Design review of the part built by this model. Coordinates are the model's own, in mm. Face numbers are marked on the shaded views. A direction names the side the tool comes from. Coordinates: 2 decimals unless noted, no trailing zeros. Loops run counter-clockwise (first coordinate to the right, second up) from the corner with the lowest first, then second, coordinate; pieces in that order, holes last. Notation, with made-up numbers: (78, 52) - (112, 52) arc R21 ccw to (112, 62) - close; hole circle Ø9 at (32, 72.5). An arc over 180 degrees is marked (long way). Answer in a Markdown table with one row per item. Add a question column.
(1) The part is to be moulded in two halves that separate along Y. For the marked faces 6, 7 and 8, say which applies: released by +Y, released by -Y, zero draft, split by the parting line, or undercut.
(2) For the marked faces 1, 2, 3, 4 and 5, list the 3-axis set-ups (+Z, -Z, +X, -X, +Y, -Y) from which the entire face can be reached by the end or side of a thin tool; tool diameter is ignored.
(3) Clearance check with flat-ended pins moving along their axes: pin 1 (1.9 mm diameter, centred on x = -0.5, y = 2, fed in from +Z); pin 2 (0.6 mm diameter, centred on x = 43, y = 31.5, fed in from +Z) (3 decimals); pin 3 (3.5 mm diameter, centred on x = 44.25, z = 4.625, fed in from +Y); pin 4 (1.6 mm diameter, centred on x = -4.5, y = 31.5, fed in from -Z) (3 decimals). State where each tip first meets the part, or that it passes through.
(4) We need section C-C, the plane x = 44.25. Write out the cut boundary in (y, z) (3 decimals).
(5) We need section A-A, the plane x = 31.5. Write out the cut boundary in (y, z), plus the area to 3 significant figures.
(6) We need section B-B, the plane y = 18. Write out the cut boundary in (x, z), plus the area to 3 significant figures.
(7) We need section D-D, the plane x = 9.35. Write out the cut boundary in (y, z) (3 decimals).
(8) To check wall thickness, follow L1, parallel to Z at x = 44, y = 29; L2, parallel to X at y = 30, z = 6.5; L3, parallel to Y at x = 16, z = 3.25. State the ranges of each line that lie inside material, in increasing order. Write a range as [from, to].
from build123d import *

# Parameters (mm, degrees)
SKETCH1_W                 = 40
SKETCH1_H                 = 20
BOSS_EXTRUDE1_DEPTH       = 34.4
BOSS_EXTRUDE2_DEPTH       = 2.8
SKETCH4_R                 = 6.95
BOSS_EXTRUDE3_DEPTH       = 1.7
SKETCH5_R                 = 5.075
BOSS_EXTRUDE4_DEPTH       = 0.5
SKETCH6_R                 = 2.875
BOSS_EXTRUDE5_DEPTH       = 3.25
BOSS_EXTRUDE6_DEPTH       = 0.75
SKETCH8_W                 = 20
SKETCH8_H                 = 2.5
BOSS_EXTRUDE7_DEPTH       = 6.7
SKETCH9_W                 = 20
SKETCH9_H                 = 2.5
BOSS_EXTRUDE8_DEPTH       = 6.7
CUT_EXTRUDE1_DEPTH        = 60.10101522
SKETCH11_W                = 6.15
SKETCH11_H                = 3.85
BOSS_EXTRUDE9_DEPTH       = 1
FILLET1_R                 = 0.75
FILLET2_R                 = 1.25
CHAMFER1_SIZE             = 0.75
BOSS_EXTRUDE10_DEPTH      = 0.625
BOSS_EXTRUDE10_DEPTH_BACK = 0.625


with BuildPart() as part:
    # Sketch1 → Boss-Extrude1 (new body)
    with BuildSketch(Plane(origin=(0, 0, 0), x_dir=(1, 0, 0), z_dir=(0, 1, 0))):
        with Locations((20, -10)):
            Rectangle(SKETCH1_W, SKETCH1_H)
    extrude(amount=BOSS_EXTRUDE1_DEPTH)

    # Sketch3 → Boss-Extrude2 (add)
    with BuildSketch(Plane(origin=(0, 34.4, 0), x_dir=(1, 0, 0), z_dir=(0, 1, 0))):
        with BuildLine():
            Line((12.775273712, -1.3), (32.775273712, -1.3))
            Line((32.775273712, -1.3), (32.775273712, -5.15))
            ThreePointArc((32.775273712, -5.15), (34.875273712, -10), (32.775273712, -14.85))
            Line((32.775273712, -14.85), (32.775273712, -18.7))
            Line((32.775273712, -18.7), (12.775273712, -18.7))
            ThreePointArc((12.775273712, -18.7), (0, -10), (12.775273712, -1.3))
        make_face()
    extrude(amount=BOSS_EXTRUDE2_DEPTH)

    # Sketch4 → Boss-Extrude3 (add)
    with BuildSketch(Plane(origin=(0, 37.2, 0), x_dir=(1, 0, 0), z_dir=(0, 1, 0))):
        with Locations(Location((9.35, -10, 0), (0, 0, 90))):
            Circle(SKETCH4_R)
    extrude(amount=BOSS_EXTRUDE3_DEPTH)

    # Sketch5 → Boss-Extrude4 (add)
    with BuildSketch(Plane(origin=(0, 38.9, 0), x_dir=(1, 0, 0), z_dir=(0, 1, 0))):
        with Locations(Location((9.35, -10, 0), (0, 0, 270))):
            Circle(SKETCH5_R)
    extrude(amount=BOSS_EXTRUDE4_DEPTH)

    # Sketch6 → Boss-Extrude5 (add)
    with BuildSketch(Plane(origin=(0, 39.4, 0), x_dir=(1, 0, 0), z_dir=(0, 1, 0))):
        with Locations(Location((9.35, -10, 0), (0, 0, 90))):
            Circle(SKETCH6_R)
    extrude(amount=BOSS_EXTRUDE5_DEPTH)

    # Sketch7 → Boss-Extrude6 (add)
    with BuildSketch(Plane(origin=(0, 37.2, 0), x_dir=(1, 0, 0), z_dir=(0, 1, 0))):
        with BuildLine():
            Line((32.775273712, -1.3), (32.775273712, -18.7))
            Line((32.775273712, -18.7), (20.275273712, -18.7))
            Line((20.275273712, -18.7), (20.275273712, -12.15))
            ThreePointArc((20.275273712, -12.15), (18.525273712, -10), (20.275273712, -7.85))
            Line((20.275273712, -7.85), (20.275273712, -1.3))
            Line((20.275273712, -1.3), (32.775273712, -1.3))
        make_face()
    extrude(amount=BOSS_EXTRUDE6_DEPTH)

    # Sketch8 → Boss-Extrude7 (add)
    with BuildSketch(Plane(origin=(40, 0, 0), x_dir=(0, 0, -1), z_dir=(1, 0, 0))):
        with Locations((-10, 28.95)):
            Rectangle(SKETCH8_W, SKETCH8_H)
    extrude(amount=BOSS_EXTRUDE7_DEPTH)

    # Sketch9 → Boss-Extrude8 (add)
    with BuildSketch(Plane.ZY):
        with Locations((10, 28.95)):
            Rectangle(SKETCH9_W, SKETCH9_H)
    extrude(amount=BOSS_EXTRUDE8_DEPTH)

    # Sketch10 → Cut-Extrude1 (cut, through all)
    with BuildSketch(Plane(origin=(0, 30.2, 0), x_dir=(1, 0, 0), z_dir=(0, 1, 0))):
        with BuildLine():
            Line((45.79029218, -3.125), (46.7, -3.125))
            Line((46.7, -3.125), (46.7, -6.125))
            Line((46.7, -6.125), (45.79029218, -6.125))
            ThreePointArc((45.79029218, -6.125), (42.1, -4.625), (45.79029218, -3.125))
        make_face()
        with BuildLine():
            Line((45.79029218, -13.875), (46.7, -13.875))
            Line((46.7, -13.875), (46.7, -16.875))
            Line((46.7, -16.875), (45.79029218, -16.875))
            ThreePointArc((45.79029218, -16.875), (42.1, -15.375), (45.79029218, -13.875))
        make_face()
        with BuildLine():
            Line((-5.79029218, -3.125), (-6.7, -3.125))
            Line((-6.7, -3.125), (-6.7, -6.125))
            Line((-6.7, -6.125), (-5.79029218, -6.125))
            ThreePointArc((-5.79029218, -6.125), (-2.1, -4.625), (-5.79029218, -3.125))
        make_face()
        with BuildLine():
            Line((-5.79029218, -13.875), (-6.7, -13.875))
            Line((-6.7, -13.875), (-6.7, -16.875))
            Line((-6.7, -16.875), (-5.79029218, -16.875))
            ThreePointArc((-5.79029218, -16.875), (-2.1, -15.375), (-5.79029218, -13.875))
        make_face()
    extrude(amount=-CUT_EXTRUDE1_DEPTH, mode=Mode.SUBTRACT)

    # Sketch11 → Boss-Extrude9 (add)
    with BuildSketch(Plane.ZY):
        with Locations((10, 1.925)):
            Rectangle(SKETCH11_W, SKETCH11_H)
    extrude(amount=BOSS_EXTRUDE9_DEPTH)

    # Fillet1
    fillet1_edges = [part.edges().sort_by_distance(p)[0] for p in [
        (40, 13.85, 0),
        (40, 13.85, 20),
        (0, 32.3, 0),
        (40, 32.3, 0),
        (40, 32.3, 20),
        (0, 13.85, 0),
        (0, 32.3, 20),
        (0, 13.85, 20),
    ]]
    fillet(fillet1_edges, radius=FILLET1_R)

    # Fillet2
    fillet2_edges = [part.edges().sort_by_distance(p)[0] for p in [
        (46.7, 28.95, 20),
        (46.7, 28.95, 0),
        (-6.7, 28.95, 0),
        (-6.7, 28.95, 20),
    ]]
    fillet(fillet2_edges, radius=FILLET2_R)

    # Chamfer1
    chamfer1_edges = [part.edges().sort_by_distance(p)[0] for p in [
        (0, 0, 16.1625),
        (0, 0, 3.8375),
        (20, 0, 0),
        (40, 0, 10),
        (20, 0, 20),
        (0.219669914, 0, 19.780330086),
        (39.780330086, 0, 19.780330086),
        (39.780330086, 0, 0.219669914),
        (0.219669914, 0, 0.219669914),
    ]]
    chamfer(chamfer1_edges, length=CHAMFER1_SIZE)

    # Sketch12 → Boss-Extrude10 (add, two sides: drawn at the far end of the back side and taken through both)
    with BuildSketch(Plane(origin=(0, 0, 10), x_dir=(-1, 0, 0), z_dir=(0, 0, -1)).offset(-BOSS_EXTRUDE10_DEPTH_BACK)):
        Polygon((-40, 32.2), (-46.7, 30.2), (-40, 30.2), align=None)
        Polygon((6.7, 30.2), (0, 32.2), (0, 30.2), align=None)
    extrude(amount=BOSS_EXTRUDE10_DEPTH + BOSS_EXTRUDE10_DEPTH_BACK)


solid = part.part
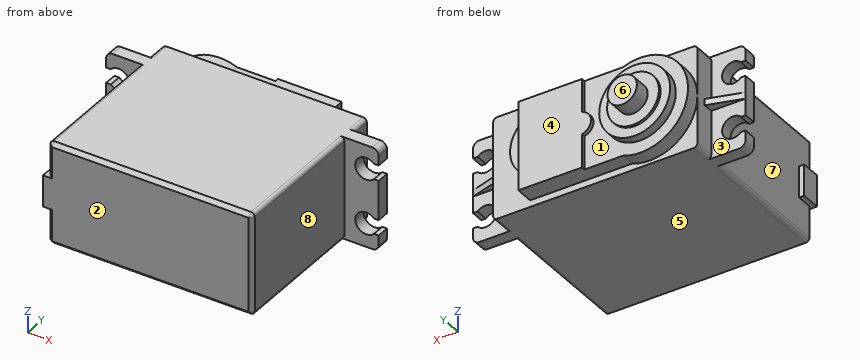
Responses:
| question | item | result |
|---|---|---|
| 1 | face 6 | released by +Y |
| 1 | face 7 | undercut |
| 1 | face 8 | zero draft |
| 2 | face 1 | +Y |
| 2 | face 2 | +Z, -Z, +X, -X, -Y |
| 2 | face 3 | -Z, -X, +Y |
| 2 | face 4 | +Z, -Z, +X, +Y |
| 2 | face 5 | -Z, +X, -X, +Y, -Y |
| 3 | pin 1 | stops at z = 19.94 |
| 3 | pin 2 | stops at z = 10.625 |
| 3 | pin 3 | passes through |
| 3 | pin 4 | stops at z = 9.375 |
| 4 | outline | (27.7, 0) - (30.2, 0) - (30.2, 2.475) - (27.7, 2.475) - close; (27.7, 6.775) - (30.2, 6.775) - (30.2, 9.375) - (30.931, 9.375) - (30.931, 10.625) - (30.2, 10.625) - (30.2, 13.225) - (27.7, 13.225) - close; (27.7, 17.525) - (30.2, 17.525) - (30.2, 20) - (27.7, 20) - close |
| 5 | outline | (0, 0.75) - (0.75, 0) - (34.4, 0) - (34.4, 1.3) - (37.95, 1.3) - (37.95, 18.7) - (34.4, 18.7) - (34.4, 20) - (0.75, 20) - (0, 19.25) - close |
| 5 | area | 749 mm2 |
| 6 | outline | (0, 0.75) arc R0.75 ccw to (0.75, 0) - (39.25, 0) arc R0.75 ccw to (40, 0.75) - (40, 19.25) arc R0.75 ccw to (39.25, 20) - (0.75, 20) arc R0.75 ccw to (0, 19.25) - close |
| 6 | area | 800 mm2 |
| 7 | outline | (0, 0.75) - (0.75, 0) - (34.4, 0) - (34.4, 0.65) - (37.2, 0.65) - (37.2, 3.05) - (38.9, 3.05) - (38.9, 4.925) - (39.4, 4.925) - (39.4, 7.125) - (42.65, 7.125) - (42.65, 12.875) - (39.4, 12.875) - (39.4, 15.075) - (38.9, 15.075) - (38.9, 16.95) - (37.2, 16.95) - (37.2, 19.35) - (34.4, 19.35) - (34.4, 20) - (0.75, 20) - (0, 19.25) - close |
| 8 | L1 | z = [0, 2.49], [6.76, 13.24], [17.51, 20] |
| 8 | L2 | x = [-6.7, -5.3], [-3.2, 43.2], [45.3, 46.7] |
| 8 | L3 | y = [0, 37.2] |
